Check sheet for the drawn part. Datum: minimum x, y, z corner. Units: mm. A direction names the side the tool comes from. Coordinates: 2 decimals unless noted, no trailing zeros. Write each loop counter-clockwise with the first axis right and the second up, starting at its lowest first coordinate (ties: lowest second). Pieces come first, ordered by that corner, then holes. Notation, with made-up numbers: (35, 47.5) -> (74, 47.5) arc R16 ccw to (74, 64.5) -> close; hole circle Ø7 at (-19, 89.25). An arc over 180 degrees is marked (long way). Answer in a Markdown table with one row per item. Add a question column.
1. Scan lines: L1, parallel to Z at x = 16.5, y = 12.25 (1 decimal); L2, parallel to Z at x = 12, y = 18; L3, parallel to Y at x = 9.5, z = 35.5. Record each from-to range of solid material in increasing order. Write a range as from..to.
2. Depth check by flat-ended pin: P1, Ø2, axis at x = 10.5, y = 9.5, coming from the +Z side; P2, Ø4, axis at x = 17, z = 23, coming from the -Y side; P3, Ø0.8, axis at x = 2.5, z = 6, coming from the +Y side. Enter the tip coordinate at first touch or a pass-through.
3. Mould release check, pull along Y, two halves, no side actions. Record for the marked faces 1, 2 and 3: pulls with the +Y half, pulls with the -Y half, needs draft (parallel to the pull), parting line crosses it, or undercut.
4. Set-up check for the marked faces 4 and 5: record each of +Z, -Z, +X, -X, +Y, -Y from which the full face is reachable in a straight line by a thin tool's end or side.
5. Cross-section at C-C on x = 16. Record the cut outline in (y, z) (1 decimal).
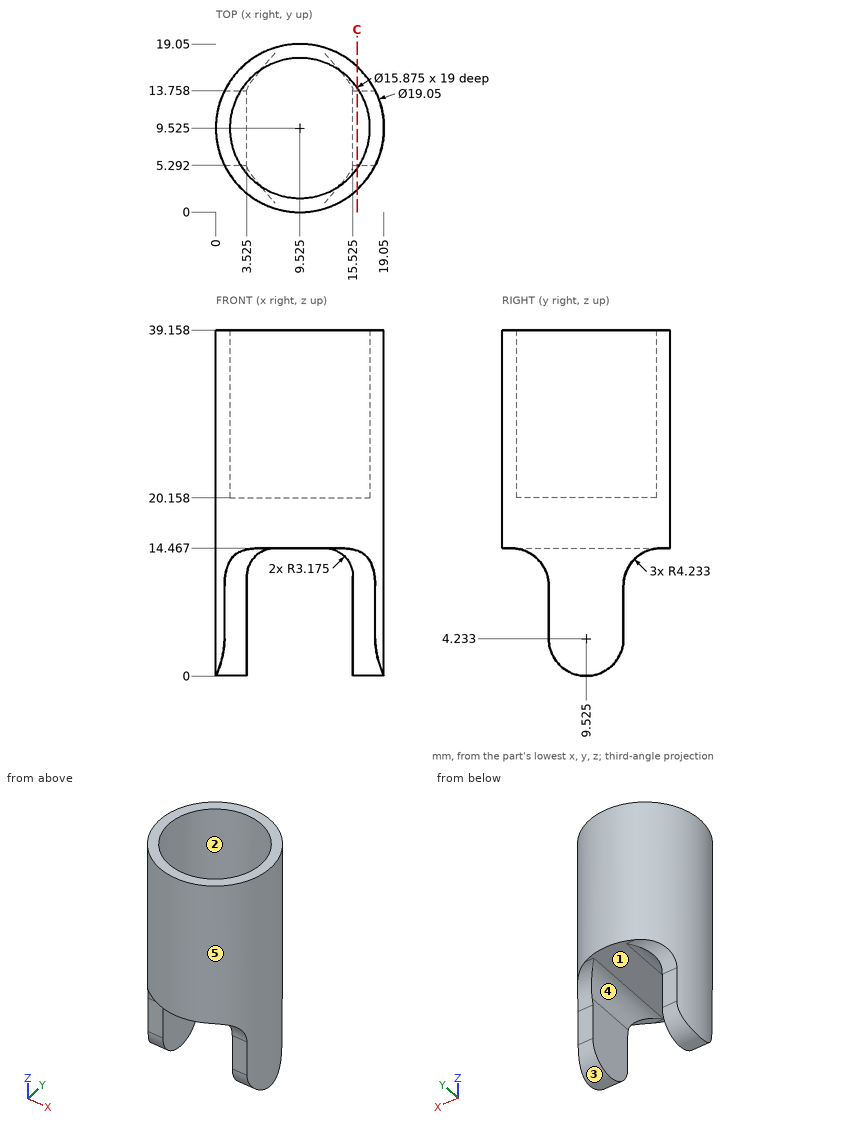
Results found:
| question | item | result |
|---|---|---|
| 1 | L1 | z = 1..20.2 |
| 1 | L2 | z = 14.47..39.16 |
| 1 | L3 | y = 0..1.59, 17.46..19.05 |
| 2 | P1 | stops at z = 20.16 |
| 2 | P2 | stops at y = 1.73 |
| 2 | P3 | stops at y = 13.76 |
| 3 | face 1 | needs draft |
| 3 | face 2 | undercut |
| 3 | face 3 | parting line crosses it |
| 4 | face 4 | -Z, +Y, -Y |
| 4 | face 5 | +Z, -Z |
| 5 | outline | (2.5, 14.2) arc R4.2 cw to (5.3, 10.2) -> (5.3, 4.2) arc R4.2 ccw to (13.8, 4.2) -> (13.8, 10.2) arc R4.2 cw to (16.5, 14.2) -> (16.5, 39.2) -> (14.1, 39.2) -> (14.1, 20.2) -> (4.9, 20.2) -> (4.9, 39.2) -> (2.5, 39.2) -> close |
